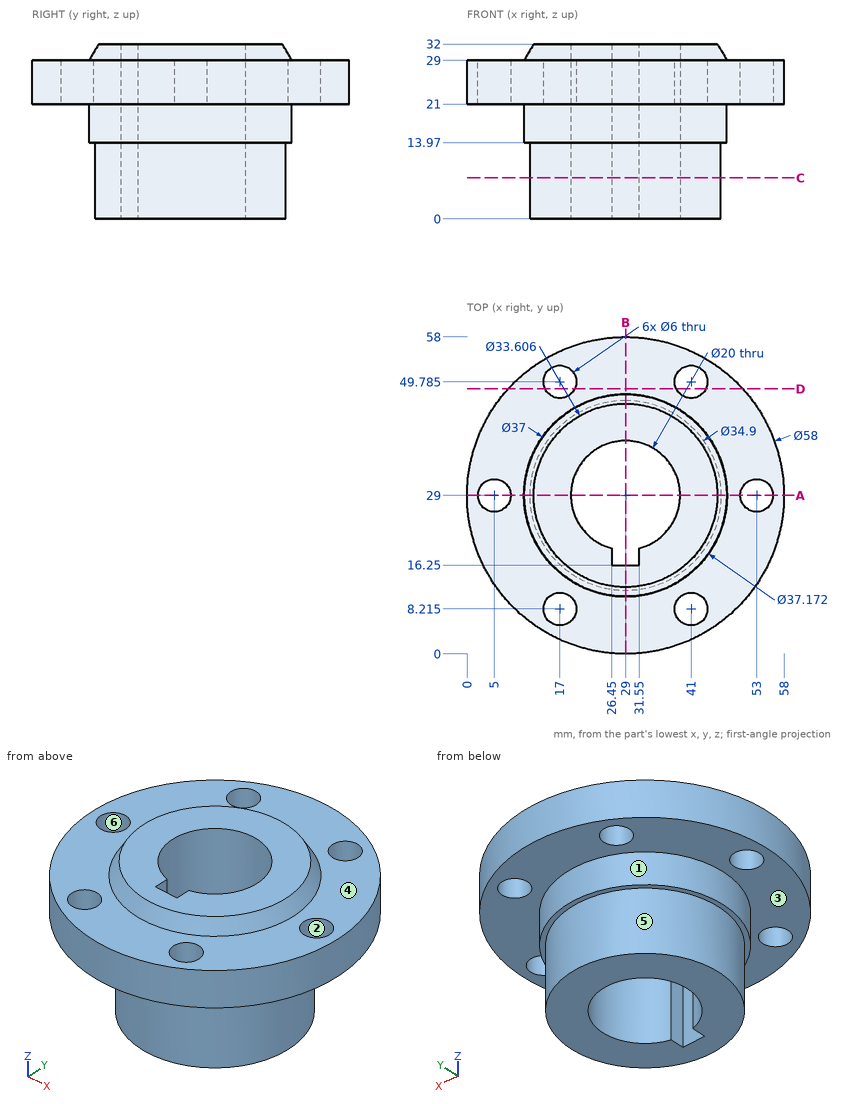
Geometry: see drawing. Coordinates: mm, zero at the bounding-box minimum. A direction names the side the tool comes from. Coordinates: 2 decimals unless noted, no trailing zeros. Loops run counter-clockwise (first coordinate to the right, second up) from the corner with the lowest first, then second, coordinate; pieces in that order, holes last.
(1) Section B-B on x = 29. Return the cut outline in (y, z), then the cut area to 3 significant figures.
(2) Section D-D on y = 48.5. Return the cut outline in (x, z) (1 decimal).
(3) Set-up query: the marked faces 4, 5 and 6. Return all of +Z, -Z, +X, -X, +Y, -Y with unobstructed straight access to the full face (end or side cutting, diameter ignored); none if empty.
(4) Pull-direction query (Y, two-part tool) for the marked faces 1, 2 and 3; classes: released by +Y, released by -Y, zero draft, split by the parting line, or undercut.
(5) Section A-A on y = 29. Return the cut outline in (x, z), then the cut area to 3 significant figures.
(6) First-contact query: pin 1 Ø7 at (x, y) = (17, 8.22) entering from +Z; pin 2 Ø4 at (y, z) = (40.5, 16) entering from -X (1 decimal); pin 3 Ø1.5 at (y, z) = (32, 3.5) entering from +X (1 decimal). Flat tips, straight axial feed; report the tip coordinate or a pass-through.
(7) Section C-C on z = 7.5. Return the cut outline in (x, y), then the cut area to 3 significant figures.
(8) Material intervals for probe 1 along X at (y, z) = (28, 23.5); probe 2 along Y at (x, z) = (41, 23) (1 decimal); probe 3 along X at (y, z) = (29.5, 9.5), sorted ascending.
Data:
1. outline: (0, 21) - (10.5, 21) - (10.5, 13.97) - (11.55, 13.97) - (11.55, 0) - (16.25, 0) - (16.25, 32) - (12.2, 32) - (10.41, 29) - (0, 29) - close; (39, 0) - (46.45, 0) - (46.45, 13.97) - (47.5, 13.97) - (47.5, 21) - (58, 21) - (58, 29) - (47.59, 29) - (45.8, 32) - (39, 32) - close
1. area: 590 mm2
2. outline: (7.5, 21) - (14.3, 21) - (14.3, 29) - (7.5, 29) - close; (19.7, 21) - (38.3, 21) - (38.3, 29) - (19.7, 29) - close; (43.7, 21) - (50.5, 21) - (50.5, 29) - (43.7, 29) - close
3. face 4: +Z
3. face 5: -Z
3. face 6: +Z, -Z
4. face 1: split by the parting line
4. face 2: undercut
4. face 3: zero draft
5. outline: (0, 21) - (2, 21) - (2, 29) - (0, 29) - close; (8, 21) - (10.5, 21) - (10.5, 13.97) - (11.55, 13.97) - (11.55, 0) - (19, 0) - (19, 32) - (12.2, 32) - (10.41, 29) - (8, 29) - close; (39, 0) - (46.45, 0) - (46.45, 13.97) - (47.5, 13.97) - (47.5, 21) - (50, 21) - (50, 29) - (47.59, 29) - (45.8, 32) - (39, 32) - close; (56, 21) - (58, 21) - (58, 29) - (56, 29) - close
5. area: 582 mm2
6. pin 1: stops at z = 29
6. pin 2: stops at x = 13.1
6. pin 3: stops at x = 46.3
7. outline: circle Ø34.9 at (29, 29); hole (26.45, 16.25) - (31.55, 16.25) - (31.55, 19.33) arc R10 ccw (long way) to (26.45, 19.33) - close
7. area: 628 mm2
8. probe 1: x = 0.02 to 2.17, 7.83 to 19.05, 38.95 to 50.17, 55.83 to 57.98
8. probe 2: y = 2.6 to 5.2, 11.2 to 46.8, 52.8 to 55.4
8. probe 3: x = 11.56 to 19.01, 38.99 to 46.44
